Design review of the part built by this model. Coordinates are the model's own, in mm. A direction names the side the tool comes from. Round coordinates to 2 decimals unless told otherwise and drop trailing zeros. Loops run counter-clockwise (first coordinate to the right, second up) from the corner with the lowest first, then second, coordinate; pieces in that order, holes last. Notation, with made-up numbers: (24.25, 19) -> (57.25, 19) arc R15 ccw to (57.25, 36) -> close; hole circle Ø2 at (-19, 89). An arc over 180 degrees is marked (long way). Answer as CSV lines item,"result". Start each with the question number.
(1) Take a section at B-B, the plane x = 33.5. Write out the cut boundary in (y, z).
(2) Take a section at C-C, the plane z = 153. Write out the cut boundary in (x, y), and give its area (3 significant figures).
(3) Draft analysis for pull direction Z (two halves, no side actions). For faces 3 (the face through (-21, 23, 101.6)), 4 (the face through (0.64, -52.914, 1.528)), 5 (the face through (24.227, 7.629, 139.186)), 6 (the face through (50.8, -1, 50)), state which applies: +Z half, -Z half, draft (parallel to the pull), parting line (faces both ways), or undercut.
(4) Machinability: for faces 1 (the face through (-49.351, -52.835, 51.44)), 2 (the face through (-25.4, -1, 52)), which of the approach directions +Z, -Z, +X, -X, +Y, -Y give a long, thin tool a straight path to every point of the face, cutting with its end or side? Answer none if there is none.
(5) Take a section at D-D, the plane z = 186. Write out the cut boundary in (x, y), and give its area (3 significant figures).
(6) Take a section at A-A, the plane y = -43. Write out the cut boundary in (x, z).
(7) For P1, Ø2, axis at y = -16, z = 162, coming from the +X side, flat-tipped, find the tip position at first contact; note if it passes through.
(8) To check wall thickness, follow line 1 (X direction, y = 4, z = 44.5); line 2 (Z direction, x = -23.5, y = 23); line 3 (Z direction, x = -20.5, y = 39.5). State the ranges of each line that lie inside material, in increasing order. Write a range as from..to.
from build123d import *

# Parameters (mm, degrees)
F0_W     = 101.6
F0_H     = 108.7252423167
F1_DEPTH = 101.6
F2_R     = 25.4
F3_DEPTH = 101.6
F8_W     = 50.8
F8_H     = 50.8
F9_DEPTH = 127
F10_R    = 5.08


with BuildPart() as f1:
    # F0 (on Top) → F1 (new body)
    with BuildSketch(Plane.XY):
        Rectangle(F0_W, F0_H)
    extrude(amount=F1_DEPTH)

    # F2 (on face) → F3 (join)
    with BuildSketch(Plane.XY.offset(101.6)):
        Circle(F2_R)
    extrude(amount=F3_DEPTH)

    # F5 (on face) → F6 (revolve)
    with BuildSketch(Plane.XY.offset(203.2)):
        with BuildLine():
            Line((0, -25.4), (0, -38.1))
            ThreePointArc((0, -38.1), (38.1, 0), (0, 38.1))
            Line((0, 38.1), (0, 25.4))
            ThreePointArc((0, 25.4), (17.9605122421, 17.9605122421), (25.4, 0))
            ThreePointArc((25.4, 0), (17.9605122421, -17.9605122421), (0, -25.4))
        make_face()
        with BuildLine():
            Line((0, 25.4), (0, -25.4))
            ThreePointArc((0, -25.4), (17.9605122421, -17.9605122421), (25.4, 0))
            ThreePointArc((25.4, 0), (17.9605122421, 17.9605122421), (0, 25.4))
        make_face()
    revolve(axis=Axis((0, 0, 203.2), (0, -1, 0)))

    # F8 (on face) → F9 (cut)
    with BuildSketch(Plane.XZ.offset(54.3626211584)):
        with Locations((0, 52.638284862)):
            Rectangle(F8_W, F8_H)
    extrude(amount=-F9_DEPTH, mode=Mode.SUBTRACT)

    # F10
    f10_edges = [f1.edges().sort_by_distance(p)[0] for p in [
        (0, -54.362621, 101.6),
        (50.8, 0, 101.6),
        (50.8, -54.362621, 50.8),
        (-50.8, 0, 101.6),
        (0, 54.362621, 101.6),
        (-50.8, -54.362621, 50.8),
        (0, -54.362621, 0),
        (50.8, 0, 0),
        (50.8, 54.362621, 50.8),
        (-50.8, 54.362621, 50.8),
        (0, 54.362621, 0),
        (-50.8, 0, 0),
        (-25.4, 0, 101.6),
        (-25.4, 0, 174.801937),
    ]]
    fillet(f10_edges, radius=F10_R)


solid = f1.part
The answers:
1,outline,"(-54.36, 5.08) arc R5.08 ccw to (-49.28, 0) -> (49.28, 0) arc R5.08 ccw to (54.36, 5.08) -> (54.36, 96.52) arc R5.08 ccw to (49.28, 101.6) -> (-49.28, 101.6) arc R5.08 ccw to (-54.36, 96.52) -> close; circle Ø36.3 at (0, 203.2)"
2,outline,"circle Ø50.8 at (0, 0)"
2,area,"2,030 mm²"
3,face 3,"undercut"
3,face 4,"-Z half"
3,face 5,"undercut"
3,face 6,"draft"
4,face 1,"+Z, -Z, -X, -Y"
4,face 2,"+Y, -Y"
5,outline,"circle Ø67.99 at (0, 0)"
5,area,"3,630 mm²"
6,outline,"(-50.8, 5.08) arc R5.08 ccw to (-45.72, 0) -> (45.72, 0) arc R5.08 ccw to (50.8, 5.08) -> (50.8, 96.52) arc R5.08 ccw to (45.72, 101.6) -> (-45.72, 101.6) arc R5.08 ccw to (-50.8, 96.52) -> close; hole (-25.4, 27.24) -> (25.4, 27.24) -> (25.4, 78.04) -> (-25.4, 78.04) -> close"
7,P1,"x = 20.5"
8,line 1,"-50.8..-25.4, 25.4..50.8"
8,line 2,"0..27.24, 78.04..101.6, 183.96..222.44"
8,line 3,"0..27.24, 78.04..101.6"
